from build123d import *

# Parameters (mm, degrees)
CROQUIS2_W              = 5
CROQUIS2_H              = 10
SALIENTE_EXTRUIR1_DEPTH = 15
CROQUIS3_R              = 1
CORTAR_EXTRUIR1_DEPTH   = 19.708286934
CROQUIS4_W              = 20
CROQUIS4_H              = 10
SALIENTE_EXTRUIR2_DEPTH = 7
CROQUIS5_W              = 2.5
CROQUIS5_H              = 6.5
CORTAR_EXTRUIR2_DEPTH   = 6
CROQUIS6_R              = 1
CORTAR_EXTRUIR3_DEPTH   = 27.162895312
CROQUIS7_W              = 2.453318502
CROQUIS7_H              = 6.5
CORTAR_EXTRUIR4_DEPTH   = 6
CROQUIS8_R              = 1
CORTAR_EXTRUIR5_DEPTH   = 27.162895312
REDONDEO1_R             = 6.5


with BuildPart() as part:
    # Croquis2 → Saliente-Extruir1 (new body)
    with BuildSketch(Plane(origin=(0, 0, 0), x_dir=(1, 0, 0), z_dir=(0, 1, 0))):
        with Locations((0, 5)):
            Rectangle(CROQUIS2_W, CROQUIS2_H)
    extrude(amount=SALIENTE_EXTRUIR1_DEPTH)

    # Croquis3 → Cortar-Extruir1 (cut, through all)
    with BuildSketch(Plane(origin=(2.5, 0, 0), x_dir=(0, 0, -1), z_dir=(1, 0, 0))):
        with Locations((5, 2.5)):
            Circle(CROQUIS3_R)
    extrude(amount=-CORTAR_EXTRUIR1_DEPTH, mode=Mode.SUBTRACT)

    # Croquis4 → Saliente-Extruir2 (add)
    with BuildSketch(Plane(origin=(0, 15, 0), x_dir=(1, 0, 0), z_dir=(0, 1, 0))):
        with Locations((-0.024823745, 5)):
            Rectangle(CROQUIS4_W, CROQUIS4_H)
    extrude(amount=SALIENTE_EXTRUIR2_DEPTH)

    # Croquis5 → Cortar-Extruir2 (cut)
    with BuildSketch(Plane.ZY.offset(10.024823745)):
        with Locations((-5, 18.75)):
            Rectangle(CROQUIS5_W, CROQUIS5_H)
    extrude(amount=-CORTAR_EXTRUIR2_DEPTH, mode=Mode.SUBTRACT)

    # Croquis6 → Cortar-Extruir3 (cut, through all)
    with BuildSketch(Plane(origin=(0, 0, -10), x_dir=(-1, 0, 0), z_dir=(0, 0, -1))):
        with Locations((8.257056792, 20.232233047)):
            Circle(CROQUIS6_R)
    extrude(amount=-CORTAR_EXTRUIR3_DEPTH, mode=Mode.SUBTRACT)

    # Croquis7 → Cortar-Extruir4 (cut)
    with BuildSketch(Plane(origin=(9.975176255, 0, 0), x_dir=(0, 0, -1), z_dir=(1, 0, 0))):
        with Locations((5, 18.75)):
            Rectangle(CROQUIS7_W, CROQUIS7_H)
    extrude(amount=-CORTAR_EXTRUIR4_DEPTH, mode=Mode.SUBTRACT)

    # Croquis8 → Cortar-Extruir5 (cut, through all)
    with BuildSketch(Plane(origin=(0, 0, -10), x_dir=(-1, 0, 0), z_dir=(0, 0, -1))):
        with Locations((-8.207409302, 20.232233047)):
            Circle(CROQUIS8_R)
    extrude(amount=-CORTAR_EXTRUIR5_DEPTH, mode=Mode.SUBTRACT)

    # Redondeo1
    # the kernel refuses this fillet: 6.5 mm, written as the material it adds along each edge
    with BuildSketch(Plane(origin=(-4.024823745, 15.5, -3.75), x_dir=(-1, 0, 0), z_dir=(0, 0, -1))) as redondeo1_piece_1:
        with BuildLine():
            CenterArc((6.5, 6.480740698), REDONDEO1_R, 180, 85.588274214)
            Line((0, 6.480740698), (-0.13, 6.480740698))
            Line((-0.13, 6.480740698), (-0.13, 0))
            Line((-0.13, 0), (0, -0.13))
            ThreePointArc((0, -0.13), (3, -0.13), (5.99, -0.129614814))
            Line((5.99, -0.129614814), (6, 0))
        make_face()
    extrude(amount=2.5)
    with BuildSketch(Plane(origin=(3.975176255, 15.5, -6.226659251), x_dir=(0, 1, 0), z_dir=(0, 0, 1))) as redondeo1_piece_2:
        with BuildLine():
            CenterArc((6.480740698, -6.5), REDONDEO1_R, 90, 85.588274214)
            Line((0, -6), (-0.129614814, -5.99))
            ThreePointArc((-0.129614814, -5.99), (-0.13, -3), (-0.13, 0))
            Line((-0.13, 0), (0, 0.13))
            Line((0, 0.13), (6.480740698, 0.13))
            Line((6.480740698, 0.13), (6.480740698, 0))
        make_face()
    extrude(amount=2.453318501)


solid = part.part
The listing builds one solid part. Answer for the finished solid, in the listing's coordinates (mm). A direction names the side the tool comes from. Coordinates: 2 decimals unless noted, no trailing zeros. Loops run counter-clockwise (first coordinate to the right, second up) from the corner with the lowest first, then second, coordinate; pieces in that order, holes last. Notation, with made-up numbers: M 28,49.25 L 71,49.25 A20 ccw 71,55.25 Z; hole C -37,5.5 d4. An arc over 180 degrees is marked long. Answer in a Markdown table with one row per item.
1) Find section C-C (z = -1). Determine the outline of the cut face in (x, y).
Answers below:
| item | result |
|---|---|
| outline | M -10.02,15 L -2.5,15 L -2.5,0 L 2.5,0 L 2.5,15 L 9.98,15 L 9.98,22 L -10.02,22 Z; hole C -8.26,20.23 d2; hole C 8.21,20.23 d2 |
2) Find section D-D (x = -8.25). Determine the outline of the cut face in (y, z), then the cut area to 3 significant figures.
Answers below:
| item | result |
|---|---|
| outline | M 15,-10 L 19.23,-10 L 19.23,-6.25 L 15.89,-6.25 L 15.89,-3.75 L 19.23,-3.75 L 19.23,0 L 15,0 Z; M 21.23,-10 L 22,-10 L 22,-6.25 L 21.23,-6.25 Z; M 21.23,-3.75 L 22,-3.75 L 22,0 L 21.23,0 Z |
| area | 39.7 mm^2 |
3) Find the intervals of material crossed by probe 1 along X at (y, z) = (10.25, -5.5); probe 2 along Y at (x, z) = (8, -1); probe 3 along Y at (x, z) = (9, -2.5), in increasing order.
Answers below:
| item | result |
|---|---|
| probe 1 | -2.5 to 2.5 |
| probe 2 | 15 to 19.25, 21.21 to 22 |
| probe 3 | 15 to 19.62, 20.84 to 22 |
4) Find section A-A (y = 2.5). Determine the outline of the cut face in (x, z).
Answers below:
| item | result |
|---|---|
| outline | M -2.5,-10 L 2.5,-10 L 2.5,-6 L -2.5,-6 Z; M -2.5,-4 L 2.5,-4 L 2.5,0 L -2.5,0 Z |
5) Given pin 1 (2.5 mm diameter, centred on y = 2.5, z = -5, fed in from -X); pin 2 (5 mm diameter, centred on y = 4.5, z = -3, fed in from +X), each flat-ended and moving along its own axis, determine where each tip first touches the part or whether it passes through.
Answers below:
| item | result |
|---|---|
| pin 1 | x = -2.5 |
| pin 2 | x = 2.5 |
6) Determine the mould class of faces 1 (the flat face through (0, 13, 0)), 2 (the flat face through (0, 0, -5)), 3 (the cylindrical face through (-5.709, 17.615, -4.982)), 4 (the flat face through (7, 19, -6.227)) for opening direction Z: released by +Z, released by -Z, zero draft, split by the parting line, or undercut.
Answers below:
| item | result |
|---|---|
| face 1 | released by +Z |
| face 2 | zero draft |
| face 3 | undercut |
| face 4 | undercut |
7) Which of the six approach directions +Z, -Z, +X, -X, +Y, -Y give full straight-line access (tool end or side, diameter ignored) to faces 5 (the cylindrical face through (5.66, 17.615, -5.017)), 6 (the flat face through (-7, 19, -6.25)), 7 (the flat face through (6, 15, -5))?
Answers below:
| item | result |
|---|---|
| face 5 | +X, +Y |
| face 6 | -X, +Y |
| face 7 | +Z, -Z, +X, -Y |
